For this review, take the finished solid that the model builds, in its own axes (mm). Face numbers are marked on the shaded views. A direction names the side the tool comes from. Round coordinates to 2 decimals unless told otherwise and drop trailing zeros. Order: outer loops, then holes, each group sorted by start corner. A loop starts at its lowest first (then second) coordinate and runs counter-clockwise, first axis right, second up. Notation, with made-up numbers: M -10.75,-27.5 L 27.25,-27.5 A20 cw 27.25,-11.5 Z; hole C 36,80 d11. An arc over 180 degrees is marked long. Answer in a Markdown table with one row per item. Add a question column.
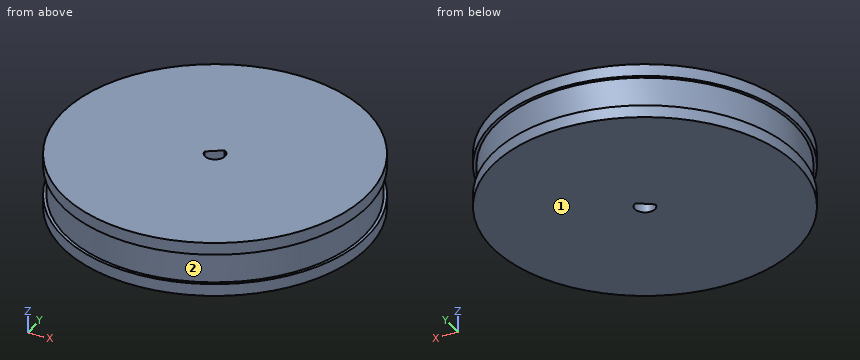
```python
from build123d import *

# Parameters (mm, degrees)
ESQUISSE1_R             = 24.5
BOSS_EXTRU_1_DEPTH      = 5
ESQUISSE2_R             = 25
BOSS_EXTRU_2_DEPTH      = 2
BOSS_EXTRU_4_START      = 2
ESQUISSE5_R             = 25
BOSS_EXTRU_4_DEPTH      = 2
ESQUISSE4_R             = 1.65
ENL_V_MAT_EXTRU_1_DEPTH = 37.482872694
BOSS_EXTRU_5_DEPTH      = 9


with BuildPart() as part:
    # Esquisse1 → Boss.-Extru.1 (new body)
    with BuildSketch(Plane.XY):
        Circle(ESQUISSE1_R)
    extrude(amount=BOSS_EXTRU_1_DEPTH)

    # Esquisse2 → Boss.-Extru.2 (add)
    with BuildSketch(Plane(origin=(0, 0, 0), x_dir=(-1, 0, 0), z_dir=(0, 0, -1))):
        Circle(ESQUISSE2_R)
    extrude(amount=BOSS_EXTRU_2_DEPTH)

    # Esquisse5 → Boss.-Extru.4 (add)
    with BuildSketch(Plane.XY.offset(5).offset(BOSS_EXTRU_4_START)):
        with Locations(Location((0, 0, 0), (0, 0, 180))):
            Circle(ESQUISSE5_R)
    extrude(amount=-BOSS_EXTRU_4_DEPTH)

    # Esquisse4 → Enlèv. mat.-Extru.1 (cut, through all)
    with BuildSketch(Plane(origin=(0, 0, -2), x_dir=(-1, 0, 0), z_dir=(0, 0, -1))):
        Circle(ESQUISSE4_R)
    extrude(amount=-ENL_V_MAT_EXTRU_1_DEPTH, mode=Mode.SUBTRACT)

    # Esquisse6 → Boss.-Extru.5 (add, through all)
    with BuildSketch(Plane.XY.offset(7)):
        with BuildLine():
            Line((-1.638440884, -0.194965301), (0.803526302, 1.441126463))
            ThreePointArc((0.803526302, 1.441126463), (-0.91840604, 1.370777278), (-1.638440884, -0.194965301))
        make_face()
    extrude(amount=-BOSS_EXTRU_5_DEPTH)


solid = part.part
```
1. Consider section D-D on y = 22.5. Write out the cut boundary in (x, z).
2. For the marked faces 1 and 2, list the 3-axis set-ups (+Z, -Z, +X, -X, +Y, -Y) from which the entire face can be reached by the end or side of a thin tool; tool diameter is ignored.
3. Consider section A-A on y = -1. Write out the cut boundary in (x, z).
4. Clearance check with flat-ended pins moving along their axes: pin 1 Ø3 at (x, y) = (0, 0) entering from -Z; pin 2 Ø1.5 at (x, z) = (-15, 3) entering from +Y; pin 3 Ø1 at (x, z) = (-15.5, 2) entering from +Y; pin 4 Ø4 at (y, z) = (-7.5, 5) entering from -X. State where each tip first meets the part, or that it passes through.
5. To check wall thickness, follow probe 1 along Y at (x, z) = (0, 2); probe 2 along X at (y, z) = (5, 4); probe 3 along X at (y, z) = (10, 4.75). State the ranges of each line that lie inside material, in increasing order. Write a range as [from, to].
6. Consider section B-B on x = -0.5. Write out the cut boundary in (y, z) (3 decimals), plus the area to 3 significant figures.
7. Consider section C-C on z = 1.25. Write out the cut boundary in (x, y), plus the area to 3 significant figures.
Solved:
| question | item | result |
|---|---|---|
| 1 | outline | M -10.9,-2 L 10.9,-2 L 10.9,0 L 9.7,0 L 9.7,5 L 10.9,5 L 10.9,7 L -10.9,7 L -10.9,5 L -9.7,5 L -9.7,0 L -10.9,0 Z |
| 2 | face 1 | -Z, +X, -X, +Y, -Y |
| 2 | face 2 | none |
| 3 | outline | M -24.98,-2 L -1.31,-2 L -1.31,7 L -24.98,7 L -24.98,5 L -24.48,5 L -24.48,0 L -24.98,0 Z; M 1.31,-2 L 24.98,-2 L 24.98,0 L 24.48,0 L 24.48,5 L 24.98,5 L 24.98,7 L 1.31,7 Z |
| 4 | pin 1 | stops at z = -2 |
| 4 | pin 2 | stops at y = 19.93 |
| 4 | pin 3 | stops at y = 19.37 |
| 4 | pin 4 | stops at x = -24.39 |
| 5 | probe 1 | y = [-24.5, -1.65], [0.9, 24.5] |
| 5 | probe 2 | x = [-23.98, 23.98] |
| 5 | probe 3 | x = [-22.37, 22.37] |
| 6 | outline | M -24.995,-2 L -1.572,-2 L -1.572,7 L -24.995,7 L -24.995,5 L -24.495,5 L -24.495,0 L -24.995,0 Z; M 0.568,-2 L 24.995,-2 L 24.995,0 L 24.495,0 L 24.495,5 L 24.995,5 L 24.995,7 L 0.568,7 Z |
| 6 | area | 426 mm^2 |
| 7 | outline | C 0,0 d49; hole M -1.64,-0.19 A1.65 ccw long 0.8,1.44 Z |
| 7 | area | 1,880 mm^2 |
